Here's how the part is built. I have some questions about the finished solid (model axes, mm). A direction names the side the tool comes from. Give positions to 0.01 mm unless a question says otherwise; leave off trailing zeros. Order: outer loops, then holes, each group sorted by start corner. A loop starts at its lowest first (then second) coordinate and runs counter-clockwise, first axis right, second up. Notation, with made-up numbers: (32, -10.75) - (78, -10.75) arc R9 ccw to (78, 5.25) - close; hole circle Ø6 at (57, 41). An arc over 180 degrees is marked (long way). One line per question, with ' | ' between items.
from build123d import *

# Parameters (mm, degrees)
IZIM2_W                        = 500
IZIM2_H                        = 300
Y_KSEKLIK_EKSTR_ZYON2_DEPTH    = 10
IZIM3_OUTSIDE_W                = 618.636
IZIM3_OUTSIDE_H                = 418.636
KES_EKSTR_ZYON1_DEPTH          = 10
TABAKLARI_UZAKLASTIRMA_2_DEPTH = 5
DAIRESEL_KAPLAMA1_COUNT        = 2
DAIRESEL_KAPLAMA1_ANGLE        = 15
AYNALAMA1_COPY_1_DEPTH         = 5
AYNALAMA1_COPY_2_DEPTH         = 5
IZIM9_R                        = 7.5
KES_EKSTR_ZYON4_DEPTH          = 8
DAIRESEL_KAPLAMA2_COUNT        = 3
IZIM10_R                       = 44
KES_EKSTR_ZYON5_DEPTH          = 5


with BuildPart() as part:
    # Çizim2 → Yükseklik-Ekstrüzyon2 (new body)
    with BuildSketch(Plane(origin=(0, 0, 0), x_dir=(1, 0, 0), z_dir=(0, 1, 0))):
        Rectangle(IZIM2_W, IZIM2_H)
    extrude(amount=Y_KSEKLIK_EKSTR_ZYON2_DEPTH)

    # Çizim3 outside → Kes-Ekstrüzyon1 (cut)
    with BuildSketch(Plane(origin=(0, 10, 0), x_dir=(1, 0, 0), z_dir=(0, 1, 0))):
        Rectangle(IZIM3_OUTSIDE_W, IZIM3_OUTSIDE_H)
        with BuildLine():
            Line((-189.1264052, 73.65761791), (205.4367974, 149.328808955))
            ThreePointArc((205.4367974, 149.328808955), (236.389117842, 141.406055572), (250, 112.5))
            Line((250, 112.5), (250, -112.5))
            ThreePointArc((250, -112.5), (236.389117842, -141.406055572), (205.4367974, -149.328808955))
            Line((205.4367974, -149.328808955), (-189.1264052, -73.65761791))
            ThreePointArc((-189.1264052, -73.65761791), (-250, 0), (-189.1264052, 73.65761791))
        make_face(mode=Mode.SUBTRACT)
    extrude(amount=-KES_EKSTR_ZYON1_DEPTH, mode=Mode.SUBTRACT)

    # Çizim6 → Tabaklari-uzaklastirma-2 (cut)
    with BuildSketch(Plane(origin=(0, 10, 0), x_dir=(1, 0, 0), z_dir=(0, 1, 0))):
        with BuildLine():
            Line((226.85, 5), (220.983294633, 5))
            ThreePointArc((220.983294633, 5), (221.340554056, 2.511336696), (221.46, 0))
            ThreePointArc((221.46, 0), (221.340554056, -2.511336696), (220.983294633, -5))
            Line((220.983294633, -5), (226.85, -5))
            Line((226.85, -5), (226.85, 5))
        make_face()
        with BuildLine():
            Line((206.85, -5), (206.85, 5))
            Line((206.85, 5), (220.983294633, 5))
            ThreePointArc((220.983294633, 5), (168.54, 0), (220.983294633, -5))
            Line((220.983294633, -5), (206.85, -5))
        make_face()
        with BuildLine():
            Line((220.983294633, 5), (206.85, 5))
            Line((206.85, 5), (206.85, -5))
            Line((206.85, -5), (220.983294633, -5))
            ThreePointArc((220.983294633, -5), (221.340554056, -2.511336696), (221.46, 0))
            ThreePointArc((221.46, 0), (221.340554056, 2.511336696), (220.983294633, 5))
        make_face()
    tabaklari_uzaklastirma_2 = extrude(amount=-TABAKLARI_UZAKLASTIRMA_2_DEPTH, mode=Mode.SUBTRACT)

    # Dairesel Kaplama1: Tabaklari-uzaklastirma-2 ×2 about axis
    dairesel_kaplama1_axis = Axis((-175, 0, 0), (0, 1, 0))
    for i in range(1, DAIRESEL_KAPLAMA1_COUNT):
        add(tabaklari_uzaklastirma_2.rotate(dairesel_kaplama1_axis, i * DAIRESEL_KAPLAMA1_ANGLE / (DAIRESEL_KAPLAMA1_COUNT - 1)), mode=Mode.SUBTRACT)

    # Aynalama1 copy 1 sketch → Aynalama1 copy 1 (cut)
    with BuildSketch(Plane(origin=(-5.962980399, 10, 45.293332893), x_dir=(0.9659258262890681, 0, 0.2588190451025214), z_dir=(0, 1, 0))):
        with BuildLine():
            Line((226.85, -5), (220.983294633, -5))
            ThreePointArc((220.983294633, -5), (221.340554056, -2.511336696), (221.46, 0))
            ThreePointArc((221.46, 0), (221.340554056, 2.511336696), (220.983294633, 5))
            Line((220.983294633, 5), (226.85, 5))
            Line((226.85, 5), (226.85, -5))
        make_face()
        with BuildLine():
            Line((206.85, 5), (206.85, -5))
            Line((206.85, -5), (220.983294633, -5))
            ThreePointArc((220.983294633, -5), (168.54, 0), (220.983294633, 5))
            Line((220.983294633, 5), (206.85, 5))
        make_face()
        with BuildLine():
            Line((220.983294633, -5), (206.85, -5))
            Line((206.85, -5), (206.85, 5))
            Line((206.85, 5), (220.983294633, 5))
            ThreePointArc((220.983294633, 5), (221.340554056, 2.511336696), (221.46, 0))
            ThreePointArc((221.46, 0), (221.340554056, -2.511336696), (220.983294633, -5))
        make_face()
    extrude(amount=-AYNALAMA1_COPY_1_DEPTH, mode=Mode.SUBTRACT)

    # Aynalama1 copy 2 sketch → Aynalama1 copy 2 (cut)
    with BuildSketch(Plane(origin=(0, 10, 0), x_dir=(1, 0, 0), z_dir=(0, 1, 0))):
        with BuildLine():
            Line((226.85, -5), (220.983294633, -5))
            ThreePointArc((220.983294633, -5), (221.340554056, -2.511336696), (221.46, 0))
            ThreePointArc((221.46, 0), (221.340554056, 2.511336696), (220.983294633, 5))
            Line((220.983294633, 5), (226.85, 5))
            Line((226.85, 5), (226.85, -5))
        make_face()
        with BuildLine():
            Line((206.85, 5), (206.85, -5))
            Line((206.85, -5), (220.983294633, -5))
            ThreePointArc((220.983294633, -5), (168.54, 0), (220.983294633, 5))
            Line((220.983294633, 5), (206.85, 5))
        make_face()
        with BuildLine():
            Line((220.983294633, -5), (206.85, -5))
            Line((206.85, -5), (206.85, 5))
            Line((206.85, 5), (220.983294633, 5))
            ThreePointArc((220.983294633, 5), (221.340554056, 2.511336696), (221.46, 0))
            ThreePointArc((221.46, 0), (221.340554056, -2.511336696), (220.983294633, -5))
        make_face()
    extrude(amount=-AYNALAMA1_COPY_2_DEPTH, mode=Mode.SUBTRACT)

    # Çizim9 → Kes-Ekstrüzyon4 (cut)
    with BuildSketch(Plane(origin=(0, 10, 0), x_dir=(1, 0, 0), z_dir=(0, 1, 0))):
        with Locations(Location((-205, 0, 0), (0, 0, 270))):
            Circle(IZIM9_R)
    kes_ekstr_zyon4 = extrude(amount=-KES_EKSTR_ZYON4_DEPTH, mode=Mode.SUBTRACT)

    # Dairesel Kaplama2: Kes-Ekstrüzyon4 ×3 about axis
    dairesel_kaplama2_axis = Axis((-175, 0, 0), (0, 1, 0))
    for i in range(1, DAIRESEL_KAPLAMA2_COUNT):
        add(kes_ekstr_zyon4.rotate(dairesel_kaplama2_axis, i * 360 / DAIRESEL_KAPLAMA2_COUNT), mode=Mode.SUBTRACT)

    # Çizim10 → Kes-Ekstrüzyon5 (cut)
    with BuildSketch(Plane(origin=(0, 10, 0), x_dir=(1, 0, 0), z_dir=(0, 1, 0))):
        with Locations(Location((-175, 0, 0), (0, 0, 270))):
            Circle(IZIM10_R)
    extrude(amount=-KES_EKSTR_ZYON5_DEPTH, mode=Mode.SUBTRACT)


solid = part.part
1) I want a section at D-D (x = 110). List the corners of the cut face in (y, z) for me.
Model answer:
outline: (0, -131.03) - (10, -131.03) - (10, 131.03) - (0, 131.03) - close
2) I want a section at B-B (x = 195). List the corners of the cut face in (y, z) for me.
Model answer:
outline: (0, -147.33) - (10, -147.33) - (10, -119.03) - (5, -119.03) - (5, -72.5) - (10, -72.5) - (10, -26.46) - (5, -26.46) - (5, 26.46) - (10, 26.46) - (10, 72.5) - (5, 72.5) - (5, 119.03) - (10, 119.03) - (10, 147.33) - (0, 147.33) - close
3) I want a section at A-A (x = -175). List the corners of the cut face in (y, z) for me.
Model answer:
outline: (0, -76.37) - (10, -76.37) - (10, -44) - (5, -44) - (5, 44) - (10, 44) - (10, 76.37) - (0, 76.37) - close
4) I'm going to push flat-ended pins straight in: P1, Ø4, axis at x = -138.5, y = 5.5, coming from the +Z side; P2, Ø5.5, axis at y = 7.5, z = 0, coming from the -X side; P3, Ø9, axis at x = -160, z = -25.98, coming from the -Y side; P4, Ø12, axis at x = -163.5, z = 26.5, coming from the +Y side. Where does each tip first touch, or does it pass through?
Model answer:
P1: stops at z = 83.75 | P2: stops at x = -250 | P3: stops at y = 0 | P4: stops at y = 5
5) Thinking about a two-plate mould opening in X: for faces 1 (the face through (52, 0, -2)), 2 (the face through (5.393, 5.07, -110.964)), 3 (the face through (-167.32, 3.52, 24.35)), 4 (the face through (250, 5, -2)), which applies, +X half, -X half, draft (parallel to the pull), parting line (faces both ways), or undercut?
Model answer:
face 1: draft | face 2: -X half | face 3: undercut | face 4: +X half
6) On a 3-axis mill with a long thin cutter (end or side, diameter ignored), from which of +Z, -Z, +X, -X, +Y, -Y can I reach the whole of each face in a straight line? I mean faces 5 (the face through (10.917, 5.07, 112.023)), 6 (the face through (168.563, 7.535, -1.093)). Say none if no direction works.
Model answer:
face 5: +Z, -X, +Y, -Y | face 6: +Y
7) Please list where these lines run through material, in increasing order: L1, parallel to X at y = 7.5, z = 10.5; L2, parallel to X at y = 4.05, z = 0; L3, parallel to Y at x = 177, z = 12.
Model answer:
L1: x = -249.26 to -217.73, -132.27 to 170.71, 219.29 to 250 | L2: x = -250 to -212.5, -197.5 to 250 | L3: y = 0 to 5
8) I want a section at C-C (z = 130). List the corners of the cut face in (x, y) for me.
Model answer:
outline: (104.65, 0) - (245.67, 0) - (245.67, 10) - (104.65, 10) - close
